from build123d import *

# Parameters (mm, degrees)
F0_R      = 15.875
F1_DEPTH  = 57.15
F2_R      = 25.4
F3_DEPTH  = 40.0558
F4_W      = 27.00502
F4_H      = 32.818373
F5_DEPTH  = 25.4
F6_W      = 22.263035
F6_H      = 30.068964
F7_DEPTH  = 25.4
F8_W      = 53.508617
F8_H      = 14.514484
F9_DEPTH  = 38.1
F11_DEPTH = 25.4
F12_W     = 57.841301
F12_H     = 15.814288
F13_DEPTH = 38.1
F15_DEPTH = 50.8


with BuildPart() as f1:
    # F0 (on Front) → F1 (new body)
    with BuildSketch(Plane.XZ):
        Circle(F0_R)
    extrude(amount=F1_DEPTH)

    # F2 (on face) → F3 (join)
    with BuildSketch(Plane.XZ.offset(57.15)):
        Circle(F2_R)
    extrude(amount=F3_DEPTH)

    # F4 (on face) → F5 (cut)
    with BuildSketch(Plane.XZ.offset(97.2058)):
        with Locations((11.89749, 16.409187)):
            Rectangle(F4_W, F4_H)
    extrude(amount=-F5_DEPTH, mode=Mode.SUBTRACT)

    # F6 (on face) → F7 (cut)
    with BuildSketch(Plane.XZ.offset(97.2058)):
        with Locations((-17.785884, -15.034482)):
            Rectangle(F6_W, F6_H)
    extrude(amount=-F7_DEPTH, mode=Mode.SUBTRACT)

    # F8 (on Right) → F9 (cut, symmetric)
    with BuildSketch(Plane.YZ):
        with Locations((-82.644399, 24.802346)):
            Rectangle(F8_W, F8_H)
    extrude(amount=F9_DEPTH, both=True, mode=Mode.SUBTRACT)

    # F10 (on face) → F11 (cut)
    with BuildSketch(Plane.YZ.offset(-1.60502)):
        Polygon((-104.001366, 21.551706), (-100.101955, 0), (-80.604888, 21.551706), align=None)
    extrude(amount=-F11_DEPTH, mode=Mode.SUBTRACT)

    # F12 (on face) → F13 (cut, symmetric)
    with BuildSketch(Plane.YZ.offset(-1.60502)):
        with Locations((-83.315812, -25.581674)):
            Rectangle(F12_W, F12_H)
    extrude(amount=F13_DEPTH, both=True, mode=Mode.SUBTRACT)

    # F14 (on face) → F15 (cut)
    with BuildSketch(Plane(origin=(-6.654367, 0, 0), x_dir=(0, -1, 0), z_dir=(-1, 0, 0))):
        Polygon((101.621397, -22.054199), (100.538224, 0), (89.923158, -22.054199), align=None)
    extrude(amount=-F15_DEPTH, mode=Mode.SUBTRACT)


solid = f1.part
The model under review builds one solid part; all positions refer to its coordinate system, in mm. A direction names the side the tool comes from. Round coordinates to 2 decimals unless told otherwise and drop trailing zeros. Order: outer loops, then holes, each group sorted by start corner. A loop starts at its lowest first (then second) coordinate and runs counter-clockwise, first axis right, second up. Notation, with made-up numbers: (78.25, -31.5) -> (129.25, -31.5) arc R26 ccw to (129.25, -16.5) -> close; hole circle Ø8 at (35.5, -23.75). An arc over 180 degrees is marked (long way). Use CSV: the item, a comma, the result in double quotes. Start each with the question number.
(1) Consider section D-D on y = -22. Write out the cut boundary in (x, z) (3 decimals), and give its area (3 significant figures).
(2) Consider section B-B on y = -79. Write out the cut boundary in (x, z), and give its area (3 significant figures).
(3) Insertion check: pin 1 (1.5 mm diameter, centred on y = -33.5, z = 5, fed in from -X); pin 2 (5.5 mm diameter, centred on y = -90, z = -5, fed in from -X); pin 3 (19.5 mm diameter, centred on y = -89, z = 13, fed in from +X) (3 decimals). Each pin has a flat end and moves straight along its axis. Give the tip position at first contact, or say it passes through.
(4) Tool access review of faces 1 (the face through (12, -71.806, 9)), 2 (the face through (-6.654, -85, -9)), 3 (the face through (-3.441, -28.175, -15.497)), 4 (the face through (8.674, -94.655, -12.224)): name each direction out of +Z, -Z, +X, -X, +Y, -Y from which nothing blocks a thin tool from reaching the whole face with its end or side.
(5) Wall thickness on probe 1 along Y at (x, z) = (22, 11.5); probe 2 along Z at (x, y) = (18, -85.5); probe 3 along Y at (x, z) = (8, 9.5): over which ranges is each line inside the solid? List them lowest first. Write a range as from..to.
(6) Consider section A-A on x = 0. Write out the cut boundary in (y, z) (3 decimals), and give its area (3 significant figures).
(7) Consider section C-C on x = 22.5. Write out the cut boundary in (y, z), and give its area (3 significant figures).
Responses:
1,outline,"circle Ø31.75 at (0, 0)"
1,area,"792 mm²"
2,outline,"(-25.4, 0) -> (-6.65, 0) -> (-6.65, -17.67) -> (18.24, -17.67) arc R25.4 ccw to (25.4, 0) -> (-1.61, 0) -> (-1.61, 17.55) -> (-18.37, 17.55) arc R25.4 ccw to start"
2,area,"906 mm²"
3,pin 1,"x = -15.3"
3,pin 2,"x = -6.65"
3,pin 3,"x = -1.605"
4,face 1,"+Z, +X, -Y"
4,face 2,"-Z, -X, -Y"
4,face 3,"+Y"
4,face 4,"-Z, +X, -X, -Y"
5,probe 1,"-71.81..-57.15"
5,probe 2,"-17.67..0"
5,probe 3,"-71.81..0"
6,outline,"(-97.206, -6.924) -> (-92.031, -17.675) -> (-57.15, -17.675) -> (-57.15, -15.875) -> (0, -15.875) -> (0, 15.875) -> (-57.15, 15.875) -> (-57.15, 17.545) -> (-71.806, 17.545) -> (-71.806, 0) -> (-97.206, 0) -> close"
6,area,"2,750 mm²"
7,outline,"(-97.21, -6.92) -> (-94.87, -11.79) -> (-57.15, -11.79) -> (-57.15, 11.79) -> (-71.81, 11.79) -> (-71.81, 0) -> (-97.21, 0) -> close"
7,area,"639 mm²"
